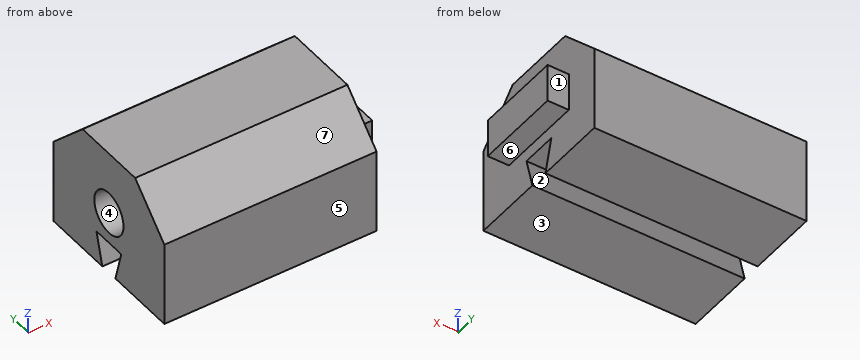
```python
from build123d import *

# Parameters (mm, degrees)
SCHIZZO1_W                   = 20.5
SCHIZZO1_H                   = 9
ESTRUSIONE_ESTRUSIONE1_DEPTH = 5
SCHIZZO2_W                   = 38
SCHIZZO2_H                   = 30
ESTRUSIONE_ESTRUSIONE2_DEPTH = 50
TAGLIO_ESTRUSIONE1_DEPTH     = 61.09159675
M8_CLEARANCE_HOLE1_D         = 10
M8_CLEARANCE_HOLE1_DEPTH     = 40
M8_CLEARANCE_HOLE1_TIP       = 3.004303095
SMUSSO1_SIZE                 = 10


with BuildPart() as part:
    # Schizzo1 → Estrusione-Estrusione1 (new body)
    with BuildSketch(Plane.YZ):
        Rectangle(SCHIZZO1_W, SCHIZZO1_H)
    extrude(amount=ESTRUSIONE_ESTRUSIONE1_DEPTH)

    # Schizzo2 → Estrusione-Estrusione2 (add)
    with BuildSketch(Plane(origin=(0, 0, 0), x_dir=(0, -1, 0), z_dir=(-1, 0, 0))):
        Rectangle(SCHIZZO2_W, SCHIZZO2_H)
    extrude(amount=ESTRUSIONE_ESTRUSIONE2_DEPTH)

    # Schizzo3 → Taglio-Estrusione1 (cut, through all)
    with BuildSketch(Plane(origin=(-50, 0, 0), x_dir=(0, -1, 0), z_dir=(-1, 0, 0))):
        Polygon((2.240381057, -15), (4.25, -7.5), (-4.25, -7.5), (-2.240381057, -15), align=None)
    extrude(amount=-TAGLIO_ESTRUSIONE1_DEPTH, mode=Mode.SUBTRACT)

    # M8 Clearance Hole1
    with Locations(Plane.ZY.offset(50)):
        with Locations((0, 0)):
            Hole(M8_CLEARANCE_HOLE1_D / 2, depth=M8_CLEARANCE_HOLE1_DEPTH)
            with Locations((0, 0, -(M8_CLEARANCE_HOLE1_DEPTH + M8_CLEARANCE_HOLE1_TIP / 2))):  # 118° drill point
                Cone(0, M8_CLEARANCE_HOLE1_D / 2, M8_CLEARANCE_HOLE1_TIP, mode=Mode.SUBTRACT)

    # Smusso1
    smusso1_edges = [part.edges().sort_by_distance(p)[0] for p in [
        (-25, -19, 15),
        (-25, 19, 15),
    ]]
    chamfer(smusso1_edges, length=SMUSSO1_SIZE)


solid = part.part
```
Part model, mm, in its own coordinate system. Face numbers are marked on the shaded views. A direction names the side the tool comes from. Round coordinates to 2 decimals unless told otherwise and drop trailing zeros. Loops run counter-clockwise (first coordinate to the right, second up) from the corner with the lowest first, then second, coordinate; pieces in that order, holes last. Notation, with made-up numbers: (45, 69) -> (104, 69) arc R22 ccw to (104, 78) -> close; hole circle Ø8 at (85.25, 58.5). An arc over 180 degrees is marked (long way). Use CSV: the item, a comma, the result in double quotes. Start each with the question number.
1) Drop flat-ended pins along their axis: P1, Ø5, axis at x = -5, z = 5.5, coming from the -Y side; P2, Ø1.5, axis at x = 2, z = 0.5, coming from the -Y side; P3, Ø5, axis at y = 8, z = -10.5, coming from the +X side; P4, Ø5.5, axis at x = 3, z = 0, coming from the +Y side. Give the stop position or say it passes through.
2) Which spindle directions (+Z, -Z, +X, -X, +Y, -Y) get a long thin tool onto all of the face, cutting with end or side? Do the marked faces 1, 2 and 3. Say none if no direction does.
3) Cut at B-B, the plane y = 6. Write the cut outline in (x, z).
4) Cut at D-D, the plane z = 10.25. Write the cut outline in (x, y).
5) Cut at A-A, the plane x = -45. Write the cut outline in (y, z).
6) Cut at C-C, the plane z = -11.75. Write the cut outline in (x, y).
7) Pull direction Z, two halves, no side cores. Call the marked faces 4, 5, 6 and 7: +Z half, -Z half, draft (parallel to the pull), parting line (faces both ways), or undercut.
8) Wall check: L1, parallel to Z at x = -35, y = 0; L2, parallel to Y at x = -39.5, z = 0; L3, parallel to X at y = -16, z = -4.5. Give the ranges that are in metal, low to high. Write a range as [from, to].
Determined:
1,P1,"stops at y = -19"
1,P2,"stops at y = -10.25"
1,P3,"stops at x = 0"
1,P4,"stops at y = 10.25"
2,face 1,"+Z, -Z, +X, +Y"
2,face 2,"+X, -X"
2,face 3,"-Z, +X, -X, +Y, -Y"
3,outline,"(-50, -15) -> (0, -15) -> (0, -4.5) -> (5, -4.5) -> (5, 4.5) -> (0, 4.5) -> (0, 15) -> (-50, 15) -> close"
4,outline,"(-50, -13.75) -> (0, -13.75) -> (0, 13.75) -> (-50, 13.75) -> close"
5,outline,"(-19, -15) -> (-2.24, -15) -> (-4.25, -7.5) -> (4.25, -7.5) -> (2.24, -15) -> (19, -15) -> (19, 5) -> (9, 15) -> (-9, 15) -> (-19, 5) -> close; hole circle Ø10 at (0, 0)"
6,outline,"(-50, -19) -> (0, -19) -> (0, -3.11) -> (-50, -3.11) -> close; (-50, 3.11) -> (0, 3.11) -> (0, 19) -> (-50, 19) -> close"
7,face 4,"undercut"
7,face 5,"draft"
7,face 6,"-Z half"
7,face 7,"+Z half"
8,L1,"z = [-7.5, -5], [5, 15]"
8,L2,"y = [-19, -5], [5, 19]"
8,L3,"x = [-50, 0]"
